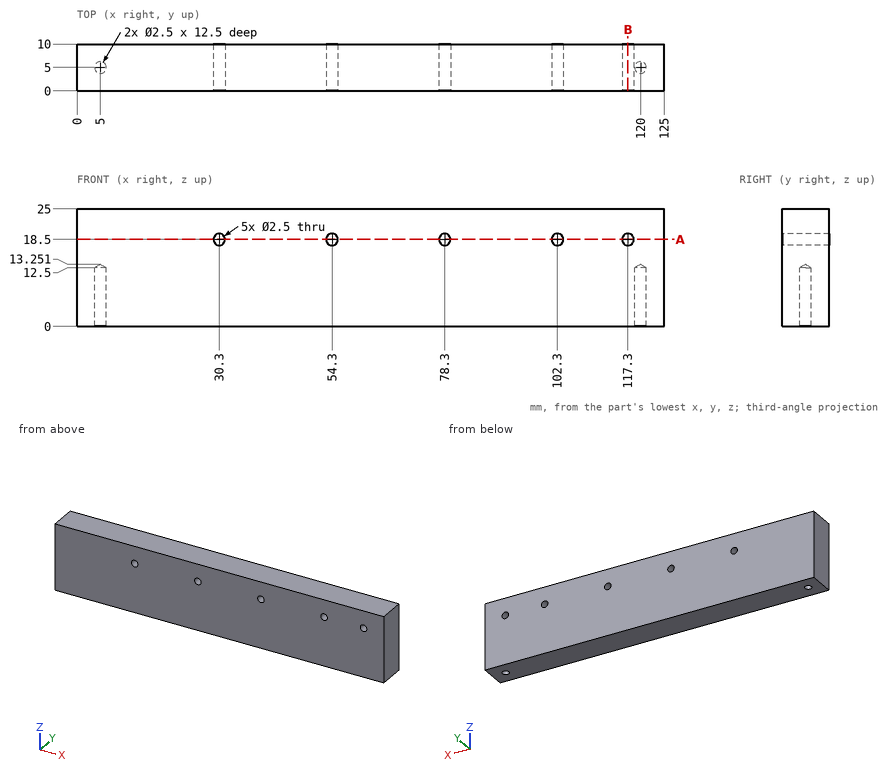
Study the drawing (mm; zero at the part's minimum x, y, z) and answer. Give positions to 0.01 mm unless a question says otherwise; leave off trailing zeros. Order: outer loops, then holes, each group sorted by start corner. A loop starts at its lowest first (then second) coordinate and runs counter-clockwise, first axis right, second up. Notation, with made-up numbers: (-34, -23.5) - (13, -23.5) arc R9 cw to (13, -7.5) - close; hole circle Ø8 at (34.5, 12.5). An arc over 180 degrees is marked (long way). Answer in a Markdown table with one row per item. Add a question column.
Q1. The part is cut by section A-A (z = 18.5). Determine the outline of the cut face in (x, y).
Q2. The part is cut by section B-B (x = 117.3). Determine the outline of the cut face in (y, z).
Q3. Find the intervals of material crossed by line 1 along X through (y, z) = (5, 9.25); line 2 along Z through (x, y) = (102.3, 7.25); line 3 along X through (y, z) = (2, 17.75), in increasing order. Write a range as [from, to].
Q4. Given P1, Ø2, axis at x = 78.3, z = 18.5, coming from the +Y side, flat-ended and moving along its own axis, determine where the tip first touches the part or whether it passes through.
Determined:
| question | item | result |
|---|---|---|
| 1 | outline | (0, 0) - (29.05, 0) - (29.05, 10) - (0, 10) - close; (31.55, 0) - (53.05, 0) - (53.05, 10) - (31.55, 10) - close; (55.55, 0) - (77.05, 0) - (77.05, 10) - (55.55, 10) - close; (79.55, 0) - (101.05, 0) - (101.05, 10) - (79.55, 10) - close; (103.55, 0) - (116.05, 0) - (116.05, 10) - (103.55, 10) - close; (118.55, 0) - (125, 0) - (125, 10) - (118.55, 10) - close |
| 2 | outline | (0, 0) - (10, 0) - (10, 17.25) - (0, 17.25) - close; (0, 19.75) - (10, 19.75) - (10, 25) - (0, 25) - close |
| 3 | line 1 | x = [0, 3.75], [6.25, 118.75], [121.25, 125] |
| 3 | line 2 | z = [0, 17.25], [19.75, 25] |
| 3 | line 3 | x = [0, 29.3], [31.3, 53.3], [55.3, 77.3], [79.3, 101.3], [103.3, 116.3], [118.3, 125] |
| 4 | P1 | passes through |
